Design review of the part built by this model. Coordinates are the model's own, in mm. A direction names the side the tool comes from. Coordinates: 2 decimals unless noted, no trailing zeros. Loops run counter-clockwise (first coordinate to the right, second up) from the corner with the lowest first, then second, coordinate; pieces in that order, holes last. Notation, with made-up numbers: M 70.5,-8 L 125.5,-8 A28 ccw 125.5,11 Z; hole C 9,20 d7. An arc over 180 degrees is marked long. Answer as a JSON object with one key per item and string values. Group by question number.
1. Consider section D-D (z = -13). State the section outline as (x, y) points, then the cut area to 3 significant figures.
2. Insertion check: pin 1 (4 mm diameter, centred on x = 2, y = -10, fed in from +Z); pin 2 (10 mm diameter, centred on x = 5, z = 8, fed in from +Y); pin 3 (1.5 mm diameter, centred on x = 8, y = 1, fed in from +Z); pin 4 (1.5 mm diameter, centred on x = -2.5, y = 3, fed in from -Z). Each pin has a flat end and moves straight along its axis. Give the tip position at first contact, or say it passes through.
3. Consider section C-C (z = -1.5). State the section outline as (x, y) points, then the cut area to 3 significant figures.
4. To check wall thickness, follow probe 1 along Y at (x, z) = (0, 7); probe 2 along Y at (x, z) = (-2.25, -0.5); probe 3 along Y at (x, z) = (5.5, 3.5). State the ranges of each line that lie inside material, in increasing order.
5. Consider section B-B (x = 0). State the section outline as (y, z) points, then the cut area to 3 significant figures.
6. Consider section A-A (y = 0). State the section outline as (x, z) points, then the cut area to 3 significant figures.
7. Draft analysis for pull direction Y (two halves, no side actions). For faces 1 (the flat face through (4, -3, 15)), 2 (the flat face through (0, -14, 0)), 3 (the flat face through (0, -13.5, 0)), state which applies: +Y half, -Y half, draft (parallel to the pull), parting line (faces both ways), or undercut.
8. Machinability: for faces 4 (the flat face through (4.88, -11.65, 0.15)), 5 (the cylindrical face through (0.1, -10.5, 0.2)), 6 (the flat face through (-4.85, -11.58, 0.15)), which of the approach directions +Z, -Z, +X, -X, +Y, -Y give a long, thin tool a straight path to every point of the face, cutting with its end or side? Answer none if there is none.
from build123d import *

# Parameters (mm, degrees)
SKETCH1_R           = 10
BOSS_EXTRUDE1_DEPTH = 15
CHAMFER1_SIZE       = 4
SKETCH2_R           = 3.75
CUT_EXTRUDE1_DEPTH  = 34.166247904
CHAMFER2_SIZE       = 1
BOSS_EXTRUDE2_DEPTH = 22


with BuildPart() as part:
    # Sketch1 → Boss-Extrude1 (new, symmetric)
    with BuildSketch(Plane.XY):
        Circle(SKETCH1_R)
    extrude(amount=BOSS_EXTRUDE1_DEPTH, both=True)

    # Chamfer1
    chamfer1_edges = [part.edges().sort_by_distance(p)[0] for p in [
        (-10, 0, -15),
        (-10, 0, 15),
    ]]
    chamfer(chamfer1_edges, length=CHAMFER1_SIZE)

    # Sketch2 → Cut-Extrude1 (cut, through all)
    with BuildSketch(Plane.XY.offset(15)):
        Circle(SKETCH2_R)
    extrude(amount=-CUT_EXTRUDE1_DEPTH, mode=Mode.SUBTRACT)

    # Chamfer2
    chamfer2_edges = [part.edges().sort_by_distance(p)[0] for p in [
        (-3.75, 0, -15),
        (-3.75, 0, 15),
    ]]
    chamfer(chamfer2_edges, length=CHAMFER2_SIZE)

    # Sketch3 → Boss-Extrude2 (add)
    with BuildSketch(Plane.XY.offset(11)):
        with BuildLine():
            Line((-3.862549243, -9.223920714), (-5.862549243, -14))
            Line((-5.862549243, -14), (5.862549243, -14))
            Line((5.862549243, -14), (3.862549243, -9.223920714))
            ThreePointArc((3.862549243, -9.223920714), (0, -10), (-3.862549243, -9.223920714))
        make_face()
        with BuildLine():
            Line((-3.589879787, -9.867257122), (-5.111103644, -13.5))
            Line((-5.111103644, -13.5), (5.111103644, -13.5))
            Line((5.111103644, -13.5), (3.589879787, -9.867257122))
            ThreePointArc((3.589879787, -9.867257122), (0, -10.5), (-3.589879787, -9.867257122))
        make_face(mode=Mode.SUBTRACT)
    extrude(amount=-BOSS_EXTRUDE2_DEPTH)


solid = part.part
Findings below:
{
 "1": {"outline": "C 0,0 d16; hole C 0,0 d7.5", "area": "157 mm^2"},
 "2": {"pin 1": "stops at z = 12.8", "pin 2": "stops at y = 10", "pin 3": "stops at z = 13.69", "pin 4": "stops at z = -14.91"},
 "3": {"outline": "M -5.86,-14 L 5.86,-14 L 3.86,-9.22 A10 ccw long -3.86,-9.22 Z; hole M -5.11,-13.5 L 5.11,-13.5 L 3.59,-9.87 A10.5 cw -3.59,-9.87 Z; hole C 0,0 d7.5", "area": "284 mm^2"},
 "4": {"probe 1": "y = -14 to -13.5, -10.5 to -3.75, 3.75 to 10", "probe 2": "y = -14 to -13.5, -10.26 to -3, 3 to 9.74", "probe 3": "y = -14 to -13.13, -8.35 to 8.35"},
 "5": {"outline": "M -14,-11 L -13.5,-11 L -13.5,11 L -14,11 Z; M -10.5,-11 L -10,-11 L -6,-15 L -4.75,-15 L -3.75,-14 L -3.75,14 L -4.75,15 L -6,15 L -10,11 L -10.5,11 Z; M 3.75,-14 L 4.75,-15 L 6,-15 L 10,-11 L 10,11 L 6,15 L 4.75,15 L 3.75,14 Z", "area": "363 mm^2"},
 "6": {"outline": "M -10,-11 L -6,-15 L -4.75,-15 L -3.75,-14 L -3.75,14 L -4.75,15 L -6,15 L -10,11 Z; M 3.75,-14 L 4.75,-15 L 6,-15 L 10,-11 L 10,11 L 6,15 L 4.75,15 L 3.75,14 Z", "area": "341 mm^2"},
 "7": {"face 1": "draft", "face 2": "-Y half", "face 3": "undercut"},
 "8": {"face 4": "+Z, -Z, +X", "face 5": "+Z, -Z", "face 6": "+Z, -Z, -X"}
}
